Design review of the part built by this model. Coordinates are the model's own, in mm. Face numbers are marked on the shaded views. Coordinates: 2 decimals unless noted, no trailing zeros. Write each loop counter-clockwise with the first axis right and the second up, starting at its lowest first coordinate (ties: lowest second). Pieces come first, ordered by that corner, then holes. Notation, with made-up numbers: M 63,6 L 67,6 A23 cw 67,44 Z; hole C -38,54.5 d7. An arc over 180 degrees is marked long. Write item = value, one per line.
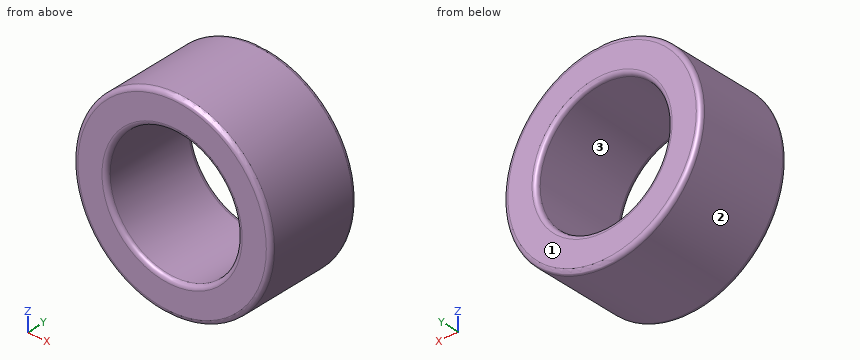
```python
from build123d import *

# Parameters (mm, degrees)
SKETCH_1_R      = 22.5
SKETCH_1_R_2    = 15
EXTRUDE_1_DEPTH = 22.5
FILLET_1_R      = 1
FILLET_2_R      = 1


with BuildPart() as part:
    # 草图1 → 凸台-拉伸1 (new body)
    with BuildSketch(Plane(origin=(0, 0, 0), x_dir=(1, 0, 0), z_dir=(0, 1, 0))):
        Circle(SKETCH_1_R)
        Circle(SKETCH_1_R_2, mode=Mode.SUBTRACT)
    extrude(amount=EXTRUDE_1_DEPTH)

    # 圆角1
    fillet_1_edges = [part.edges().sort_by_distance(p)[0] for p in [
        (-22.5, 22.5, 0),
    ]]
    fillet(fillet_1_edges, radius=FILLET_1_R)

    # 圆角2
    fillet_2_edges = [part.edges().sort_by_distance(p)[0] for p in [
        (-22.5, 0, 0),
        (-15, 0, 0),
        (-15, 22.5, 0),
    ]]
    fillet(fillet_2_edges, radius=FILLET_2_R)


solid = part.part
```
Q1. The part is to be moulded in two halves that separate along X. For the marked faces 1, 2 and 3, say which applies: +X half, -X half, draft (parallel to the pull), parting line (faces both ways), or undercut.
Check result:
face_1 = draft
face_2 = parting line
face_3 = undercut
Q2. Consider section C-C, the plane y = 15.5. State the section outline as (x, z) points.
Check result:
outline = C 0,0 d45; hole C 0,0 d30
Q3. For P1, Ø1.5, axis at y = 4.5, z = 9.5, coming from the +X side; P2, Ø4, axis at x = 0.5, y = 17.5, coming from the -Z side; P3, Ø1, axis at x = 18, y = 4.5, coming from the -Z side, all flat-tipped, find the tip position at first contact; note any pin that passes through.
Check result:
P1 = 20.73
P2 = -22.5
P3 = -14.14
Q4. Consider section A-A, the plane z = 0. State the section outline as (x, y) points.
Check result:
outline = M -22.5,1 A1 ccw -21.5,0 L -16,0 A1 ccw -15,1 L -15,21.5 A1 ccw -16,22.5 L -21.5,22.5 A1 ccw -22.5,21.5 Z; M 15,1 A1 ccw 16,0 L 21.5,0 A1 ccw 22.5,1 L 22.5,21.5 A1 ccw 21.5,22.5 L 16,22.5 A1 ccw 15,21.5 Z
Q5. Wall thickness on line 1 (Z direction, x = 0, y = 16.25); line 2 (Z direction, x = -4, y = 9.75): over which ranges is each line inside the solid? List them lowest first.
Check result:
line_1 = -22.5 to -15, 15 to 22.5
line_2 = -22.14 to -14.46, 14.46 to 22.14
Q6. Consider section B-B, the plane x = 0. State the section outline as (y, z) points.
Check result:
outline = M 0,-21.5 A1 ccw 1,-22.5 L 21.5,-22.5 A1 ccw 22.5,-21.5 L 22.5,-16 A1 ccw 21.5,-15 L 1,-15 A1 ccw 0,-16 Z; M 0,16 A1 ccw 1,15 L 21.5,15 A1 ccw 22.5,16 L 22.5,21.5 A1 ccw 21.5,22.5 L 1,22.5 A1 ccw 0,21.5 Z
